Model file for the job. Use its own axes, mm. Face numbers are marked on the shaded views. Coordinates: 2 decimals unless noted, no trailing zeros. Order: outer loops, then holes, each group sorted by start corner. A loop starts at its lowest first (then second) coordinate and runs counter-clockwise, first axis right, second up. Notation, with made-up numbers: (0.25, 13) -> (11.25, 13) arc R26 cw to (11.25, 48) -> close; hole circle Ø5 at (87.5, 46.25). An arc over 180 degrees is marked (long way). Return JSON: item names as keys, results as strings. Group by question number.
1) Flat gauge pins, fed straight in: pin 1 (0.7 mm diameter, centred on y = -0.5, z = -14, fed in from +X); pin 2 (1.1 mm diameter, centred on x = -14, y = 1.5, fed in from -Z); pin 3 (1.5 mm diameter, centred on x = -11, y = -4, fed in from -Z). Where does each tip first touch, or does it go through?
2) Probe line 1 (X direction, y = -3, z = 0); line 2 (Z direction, x = 0, y = 0); line 3 (X direction, y = 3.5, z = 0). List the from-to ranges inside material, lowest first.
3) Cut at C-C (y = -5.5). Write the cut outline in (x, z), and give its area (3 significant figures).
4) Cut at B-B (x = 0). Write the cut outline in (y, z).
5) Cut at A-A (z = -4.5). Write the cut outline in (x, y), and give its area (3 significant figures).
6) Pull direction Z, two halves, no side cores. Call the marked faces 1, 2, 3 and 4: +Z half, -Z half, draft (parallel to the pull), parting line (faces both ways), or undercut.
7) Cut at D-D (z = 0.5). Write the cut outline in (x, y).
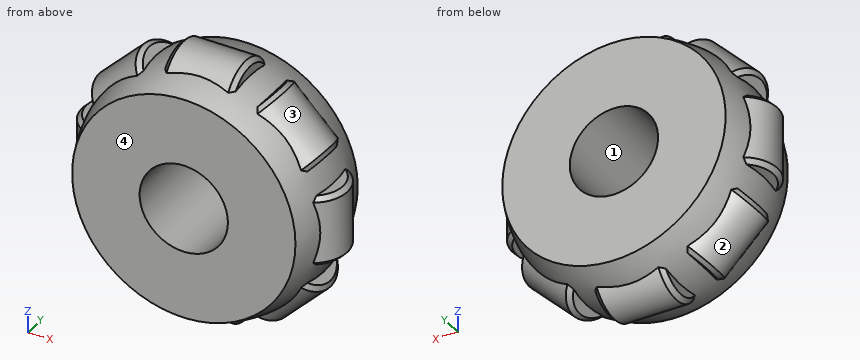
from build123d import *

# Parameters (mm, degrees)
SKETCH_3_W                           = 8
SKETCH_3_H                           = 4
CHAMFER_1_SIZE                       = 0.5
PATTERN_CIRCULAR_1_COUNT             = 8
CHAMFER_1_OF_PATTERN_CIRCULAR_1_SIZE = 0.5


with BuildPart() as part:
    # 草图5 → 旋转1 (revolve)
    with BuildSketch(Plane.XY):
        with BuildLine():
            Line((5, 6), (5, -6))
            Line((5, -6), (12.649110641, -6))
            ThreePointArc((12.649110641, -6), (14, 0), (12.649110641, 6))
            Line((12.649110641, 6), (5, 6))
        make_face()
    revolve(axis=Axis((0, 0, 0), (0, 1, 0)))

    # 草图3 → 旋转2 (revolve)
    with BuildSketch(Plane(origin=(0, 0, 0), x_dir=(1, 0, 0), z_dir=(0, 1, 0))):
        with Locations((0, 13)):
            Rectangle(SKETCH_3_W, SKETCH_3_H)
    revolve_2 = revolve(axis=Axis((-4, 0, -11), (1, 0, 0)))

    # 倒角1
    chamfer_1_edges = [part.edges().sort_by_distance(p)[0] for p in [
        (-4, 0, -15),
        (4, 0, -15),
    ]]
    chamfer(chamfer_1_edges, length=CHAMFER_1_SIZE)

    # 阵列(圆周)1: 旋转2 ×8 about axis
    pattern_circular_1_axis = Axis((0, 0, 0), (0, 1, 0))
    for i in range(1, PATTERN_CIRCULAR_1_COUNT):
        add(revolve_2.rotate(pattern_circular_1_axis, i * 360 / PATTERN_CIRCULAR_1_COUNT))

    # 倒角1 of 阵列(圆周)1
    chamfer_1_of_pattern_circular_1_edges = [part.edges().sort_by_distance(p)[0] for p in [
        (-13.435028843, 0, -7.778174593),
        (-7.778174593, 0, -13.435028843),
        (-15, 0, 4),
        (-15, 0, -4),
        (-7.778174593, 0, 13.435028843),
        (-13.435028843, 0, 7.778174593),
        (4, 0, 15),
        (-4, 0, 15),
        (13.435028843, 0, 7.778174593),
        (7.778174593, 0, 13.435028843),
        (15, 0, -4),
        (15, 0, 4),
        (7.778174593, 0, -13.435028843),
        (13.435028843, 0, -7.778174593),
    ]]
    chamfer(chamfer_1_of_pattern_circular_1_edges, length=CHAMFER_1_OF_PATTERN_CIRCULAR_1_SIZE)


solid = part.part
Answers below:
{
 "1": {"pin 1": "stops at x = 4", "pin 2": "stops at z = -4", "pin 3": "stops at z = -8.72"},
 "2": {"line 1": "x = -13.67 to -5, 5 to 13.67", "line 2": "z = -15 to -5, 5 to 15", "line 3": "x = -13.56 to -5, 5 to 13.56"},
 "3": {"outline": "circle Ø25.75 at (0, 0); hole circle Ø10 at (0, 0)", "area": "442 mm^2"},
 "4": {"outline": "(-6, -12.65) arc R14 ccw to (-2.97, -13.68) arc R4 ccw to (2.97, -13.68) arc R14 ccw to (6, -12.65) -> (6, -5) -> (-6, -5) -> close; (-6, 5) -> (6, 5) -> (6, 12.65) arc R14 ccw to (2.97, 13.68) arc R4 ccw to (-2.97, 13.68) arc R14 ccw to (-6, 12.65) -> close"},
 "5": {"outline": "(-11.82, -6) -> (-2.18, -6) -> (-2.18, 6) -> (-11.82, 6) arc R13.26 ccw to start; (2.18, -6) -> (11.82, -6) arc R13.26 ccw to (11.82, 6) -> (2.18, 6) -> close", "area": "255 mm^2"},
 "6": {"face 1": "undercut", "face 2": "-Z half", "face 3": "+Z half", "face 4": "draft"},
 "7": {"outline": "(-13.67, -2.98) arc R13.99 ccw to (-12.64, -6) -> (-4.97, -6) -> (-4.97, 6) -> (-12.64, 6) arc R13.99 ccw to (-13.67, 2.98) arc R4 ccw to start; (4.97, -6) -> (12.64, -6) arc R13.99 ccw to (13.67, -2.98) arc R4 ccw to (13.67, 2.98) arc R13.99 ccw to (12.64, 6) -> (4.97, 6) -> close"}
}
